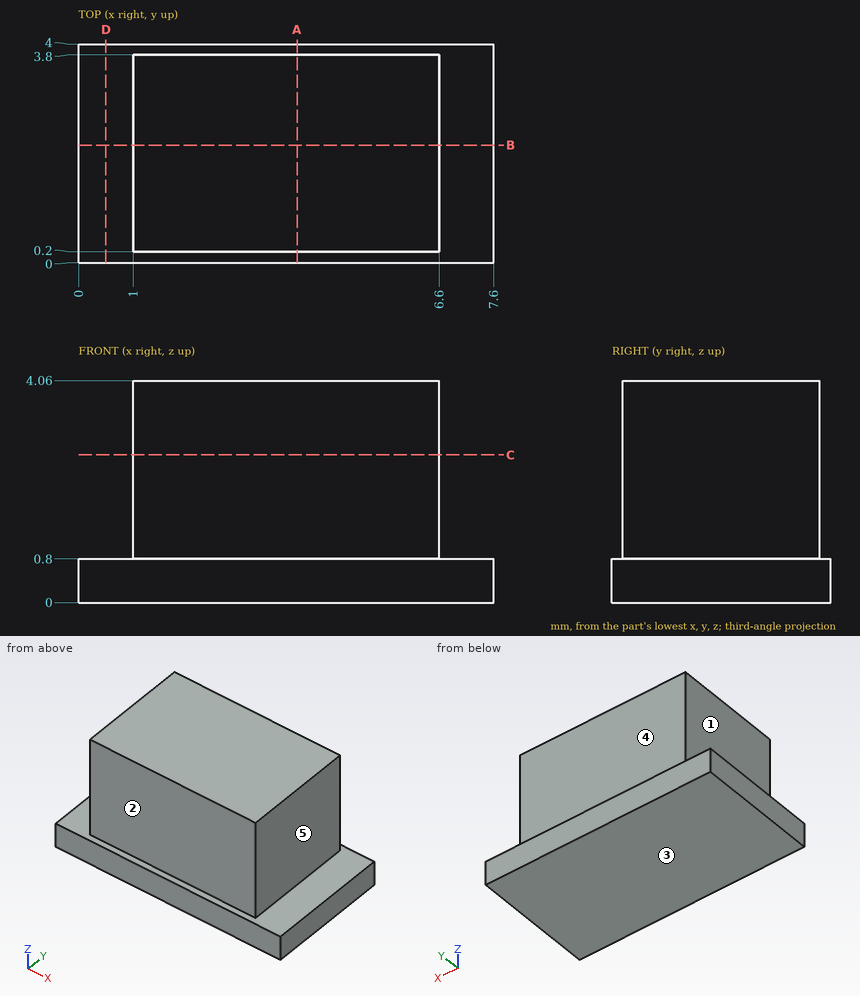
Design review of the part shown in the three views and the two pictorial views. Dimensions are in mm from the part's minimum x, y and z. A direction names the side the tool comes from. Give positions to 0.01 mm unless a question says otherwise; leave off trailing zeros. Loops run counter-clockwise (first coordinate to the right, second up) from the corner with the lowest first, then second, coordinate; pieces in that order, holes last. Notation, with made-up numbers: M 51.25,80.25 L 79.25,80.25 A23 cw 79.25,109.25 Z; hole C -30.75,16 d7. An arc over 180 degrees is marked long. Answer as a JSON object with one key per item and string values.
Item 1: We need section C-C (z = 2.7). State the section outline as (x, y) points, and give its area (3 significant figures).
Output values:
{"outline": "M 1,0.2 L 6.6,0.2 L 6.6,3.8 L 1,3.8 Z", "area": "20.2 mm2"}
Item 2: We need section D-D (x = 0.5). State the section outline as (y, z) points.
Output values:
{"outline": "M 0,0 L 4,0 L 4,0.8 L 0,0.8 Z"}
Item 3: Machinability: for the marked faces 1, 2, 3, 4 and 5, which of the approach directions +Z, -Z, +X, -X, +Y, -Y give a long, thin tool a straight path to every point of the face, cutting with its end or side? Answer none if there is none.
Output values:
{"face 1": "+Z, -X, +Y, -Y", "face 2": "+Z, +X, -X, -Y", "face 3": "-Z, +X, -X, +Y, -Y", "face 4": "+Z, +X, -X, +Y", "face 5": "+Z, +X, +Y, -Y"}
Item 4: We need section A-A (x = 4). State the section outline as (y, z) points, and give its area (3 significant figures).
Output values:
{"outline": "M 0,0 L 4,0 L 4,0.8 L 3.8,0.8 L 3.8,4.06 L 0.2,4.06 L 0.2,0.8 L 0,0.8 Z", "area": "14.9 mm2"}
Item 5: For P1, Ø1.5, axis at y = 1.5, z = 2.5, coming from the +X side; P2, Ø2, axis at x = 5.5, z = 2.5, coming from the -Y side; P3, Ø1, axis at y = 1.5, z = 2.5, coming from the -X side, all flat-tipped, find the tip position at first contact; note any pin that passes through.
Output values:
{"P1": "stops at x = 6.6", "P2": "stops at y = 0.2", "P3": "stops at x = 1"}
Item 6: Wall thickness on line 1 along X through (y, z) = (1.7, 1.8); line 2 along Y through (x, z) = (5.5, 1.85); line 3 along Z through (x, y) = (7, 2.05): over which ranges is each line inside the solid? List them lowest first.
Output values:
{"line 1": "x = 1 to 6.6", "line 2": "y = 0.2 to 3.8", "line 3": "z = 0 to 0.8"}
Item 7: We need section B-B (y = 2.15). State the section outline as (x, z) points, and give its area (3 significant figures).
Output values:
{"outline": "M 0,0 L 7.6,0 L 7.6,0.8 L 6.6,0.8 L 6.6,4.06 L 1,4.06 L 1,0.8 L 0,0.8 Z", "area": "24.3 mm2"}
